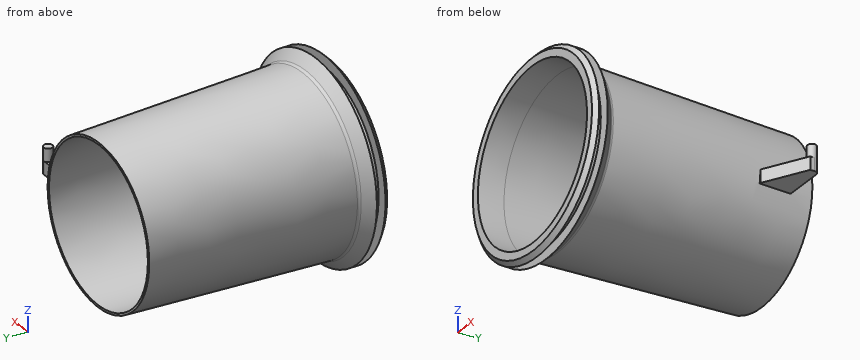
```python
from build123d import *

# Parameters (mm, degrees)
BOSS_EXTRUDE1_DEPTH = 3
BOSS_EXTRUDE2_START = 3
SKETCH2_3_R         = 1
BOSS_EXTRUDE2_DEPTH = 3


with BuildPart() as part:
    # Sketch1 → Revolve1 (revolve)
    with BuildSketch(Plane.XY):
        with BuildLine():
            Line((19.500030777, 2.904604688), (19.706224116, -3))
            Line((19.706224116, -3), (21.5, -3))
            Line((21.5, -3), (22.5, -2))
            Line((22.5, -2), (20, -2))
            Line((20, -2), (20, 0))
            Line((20, 0), (22.5, 0))
            Line((22.5, 0), (20.292893219, 2.207106781))
            ThreePointArc((20.292893219, 2.207106781), (20.076120467, 2.53153013), (20, 2.914213562))
            Line((20, 2.914213562), (18.355728105, 50))
            Line((18.355728105, 50), (17.856032692, 50))
            Line((17.856032692, 50), (17.856032692, 49.982550252))
            Line((17.856032692, 49.982550252), (19.500030777, 2.904604688))
        make_face()
    revolve(axis=Axis((0, 0, 0), (0, 1, 0)))

    # Sketch2 → Boss-Extrude1 (add)
    with BuildSketch(Plane.XY):
        with BuildLine():
            Line((18.285809554, 37.684078697), (18.785809554, 37.684078697))
            Line((18.785809554, 37.684078697), (28.530331953, 43))
            Line((28.530331953, 43), (28.530331953, 44))
            ThreePointArc((28.530331953, 44), (28.237438734, 44.707106781), (27.530331953, 45))
            Line((27.530331953, 45), (18.285809554, 45))
            Line((18.285809554, 45), (18.285809554, 37.684078697))
        make_face()
    extrude(amount=-BOSS_EXTRUDE1_DEPTH)

    # Sketch2_3 → Boss-Extrude2 (add)
    with BuildSketch(Plane.XY.offset(BOSS_EXTRUDE2_START)):
        with Locations((27.530331953, 44)):
            Circle(SKETCH2_3_R)
    extrude(amount=-BOSS_EXTRUDE2_DEPTH)


solid = part.part
```
For this review, take the finished solid that the model builds, in its own axes (mm). Give positions to 0.01 mm unless a question says otherwise; leave off trailing zeros. Write each loop counter-clockwise with the first axis right and the second up, starting at its lowest first coordinate (ties: lowest second). Pieces come first, ordered by that corner, then holes. Notation, with made-up numbers: M 44,56 L 91,56 A25 cw 91,90 Z; hole C 9.5,55 d9. An arc over 180 degrees is marked long. Answer as a JSON object with one key per item and string values. Group by question number.
Item 1: Consider section A-A on y = 30. Write out the cut boundary in (x, z), plus the area to 3 significant figures.
Item 2: For probe 1 along Z at (x, y) = (7.5, 36); probe 2 along Z at (x, y) = (-1, 16); probe 3 along X at (y, z) = (20.5, 4), list the stretches that pass through material, from the lowest coordinate up. Write a range as [from, to].
Item 3: For pin 1 Ø1.5 at (x, y) = (2, 35) entering from +Z; pin 2 Ø4 at (x, y) = (17, 22) entering from +Z; pin 3 Ø1.6 at (x, y) = (27.5, 44) entering from +Z, all flat-tipped, find the tip position at first contact; note any pin that passes through.
Item 4: Consider section B-B on y = 18. Write out the cut boundary in (x, z), plus the area to 3 significant figures.
Check result:
{
 "1": {"outline": "C 0,0 d38.11; hole C 0,0 d37.11", "area": "59.1 mm^2"},
 "2": {"probe 1": "z = [-17.29, -16.74], [16.74, 17.29]", "probe 2": "z = [-19.52, -19.02], [19.02, 19.52]", "probe 3": "x = [-18.97, -18.46], [18.46, 18.97]"},
 "3": {"pin 1": "stops at z = 18.84", "pin 2": "stops at z = 12.2", "pin 3": "stops at z = 3"},
 "4": {"outline": "C 0,0 d38.95; hole C 0,0 d37.95", "area": "60.4 mm^2"}
}
